```python
from build123d import *

# Parameters (mm, degrees)
F1_DEPTH        = 66
F2_R            = 7.5
F3_DEPTH        = 19.501
F5_DEPTH        = 6
F7_DEPTH        = 13.5
F8_R            = 1.5
F9_DEPTH        = 6.001
F11_D           = 3
F11_CSINK_D     = 7.5
F11_CSINK_ANGLE = 90


with BuildPart() as f1:
    # F0 (on Front) → F1 (new body)
    with BuildSketch(Plane.XZ):
        Polygon((0, 70), (0, 0), (19.5, 0), (19.5, 25), (6, 25), (6, 70), align=None)
    extrude(amount=F1_DEPTH)

    # F2 (on face) → F3 (cut, through all)
    with BuildSketch(Plane.YZ.offset(19.5)):
        with Locations((-9.5, 16)):
            Circle(F2_R)
    extrude(amount=-F3_DEPTH, mode=Mode.SUBTRACT)

    # F4 (on face) → F5 (cut)
    with BuildSketch(Plane.YZ.offset(19.5)):
        with BuildLine():
            Line((0, 25), (-20.223805, 25))
            ThreePointArc((-20.223805, 25), (-19.161138, 5.867754), (0, 5.716518))
            Line((0, 5.716518), (0, 25))
        make_face()
    extrude(amount=-F5_DEPTH, mode=Mode.SUBTRACT)

    # F6 (on face) → F7 (cut)
    with BuildSketch(Plane.YZ.offset(19.5)):
        Polygon((-3.5, 25), (0, 21.5), (0, 25), align=None)
    extrude(amount=-F7_DEPTH, mode=Mode.SUBTRACT)

    # F8 (on face) → F9 (cut, through all)
    with BuildSketch(Plane.YZ.offset(6)):
        with Locations((-17.5, 82.5)):
            Circle(F8_R)
        with Locations((-48.5, 82.5)):
            Circle(F8_R)
    extrude(amount=-F9_DEPTH, mode=Mode.SUBTRACT)

    # F11 (through all)
    with Locations(Plane(origin=(0, 0, 0), x_dir=(0, -1, 0), z_dir=(-1, 0, 0))):
        with Locations((31, 12.5), (56, 12.5), (56, 12.5)):
            CounterSinkHole(F11_D / 2, F11_CSINK_D / 2, counter_sink_angle=F11_CSINK_ANGLE)


solid = f1.part
```
The listing builds one solid part. Answer for the finished solid, in the listing's coordinates (mm). A direction names the side the tool comes from. Coordinates: 2 decimals unless noted, no trailing zeros. Loops run counter-clockwise (first coordinate to the right, second up) from the corner with the lowest first, then second, coordinate; pieces in that order, holes last. Notation, with made-up numbers: (-15.5, 79) -> (27.5, 79) arc R19 cw to (27.5, 107) -> close; hole circle Ø5 at (23, 67). An arc over 180 degrees is marked (long way). Return JSON: item names as keys, results as strings. Group by question number.
(1) Given pin 1 Ø13.5 at (y, z) = (-9.5, 16) entering from -X; pin 2 Ø2 at (x, y) = (15, -50.5) entering from +Z; pin 3 Ø4 at (y, z) = (-31, 12.5) entering from -X; pin 4 Ø10 at (y, z) = (-14, 31.5) entering from +X, each flat-ended and moving along its own axis, determine where each tip first touches the part or whether it passes through.
(2) A cutting plane is placed at C-C on z = 22.5. Write down the section's boundary in (x, y).
(3) A cutting plane is placed at B-B on y = -56. Write down the section's boundary in (x, z).
(4) Determine the mould class of faces 6 (the flat face through (6, -33, 45)), 7 (the cylindrical face through (11, -54.57, 12.95)), 8 (the flat face through (5, -66, 28)) for opening direction Y: released by +Y, released by -Y, zero draft, split by the parting line, or undercut.
(5) A cutting plane is placed at A-A on x = 4.25. Write down the section's boundary in (y, z), and give its area (3 significant figures).
(6) Which of the six approach directions +Z, -Z, +X, -X, +Y, -Y give full straight-line access (tool end or side, diameter ignored) to faces 1 (the cylindrical face through (11, -32.2, 11.6)), 2 (the flat face through (9.8, -1.8, 23.3)), 3 (the flat face through (13, -34, 25)), 4 (the flat face through (5, 0, 28)), 5 (the cylindrical face through (16.5, -19.4, 6.1))?
(7) Find the intervals of material crossed by probe 1 along Y at (x, z) = (3.5, 16.5); probe 2 along Z at (x, y) = (3.5, -31); probe 3 along Z at (x, y) = (9, -9.5), in increasing order. Write a range as from..to.
(8) A cutting plane is placed at D-D on z = 12.5. Write down the section's boundary in (x, y).
The answers:
{
 "1": {"pin 1": "passes through", "pin 2": "stops at z = 25", "pin 3": "stops at x = 1.75", "pin 4": "stops at x = 6"},
 "2": {"outline": "(0, -66) -> (19.5, -66) -> (19.5, -21.9) -> (13.5, -21.9) -> (13.5, -13.24) -> (0, -13.24) -> close; (0, -5.76) -> (13.5, -5.76) -> (13.5, -1) -> (6, -1) -> (6, 0) -> (0, 0) -> close"},
 "3": {"outline": "(0, 0) -> (19.5, 0) -> (19.5, 11) -> (2.25, 11) -> (0, 8.75) -> close; (0, 16.25) -> (2.25, 14) -> (19.5, 14) -> (19.5, 25) -> (6, 25) -> (6, 70) -> (0, 70) -> close"},
 "4": {"face 6": "zero draft", "face 7": "undercut", "face 8": "released by -Y"},
 "5": {"outline": "(-66, 0) -> (0, 0) -> (0, 70) -> (-66, 70) -> close; hole circle Ø3 at (-56, 12.5); hole circle Ø3 at (-31, 12.5); hole circle Ø15 at (-9.5, 16)", "area": "4,430 mm^2"},
 "6": {"face 1": "+X, -X", "face 2": "+Z, +X, +Y", "face 3": "+Z, +X, +Y, -Y", "face 4": "+Z, -Z, +X, -X, +Y", "face 5": "+X"},
 "7": {"probe 1": "y = -66..-16.98, -2.02..0", "probe 2": "z = 0..11, 14..70", "probe 3": "z = 0..8.5, 23.5..25"},
 "8": {"outline": "(0, -66) -> (19.5, -66) -> (19.5, -57.5) -> (2.25, -57.5) -> (0, -59.75) -> close; (0, -52.25) -> (2.25, -54.5) -> (19.5, -54.5) -> (19.5, -32.5) -> (2.25, -32.5) -> (0, -34.75) -> close; (0, -27.25) -> (2.25, -29.5) -> (19.5, -29.5) -> (19.5, -23.06) -> (13.5, -23.06) -> (13.5, -16.13) -> (0, -16.13) -> close; (0, -2.87) -> (13.5, -2.87) -> (13.5, 0) -> (0, 0) -> close"}
}
